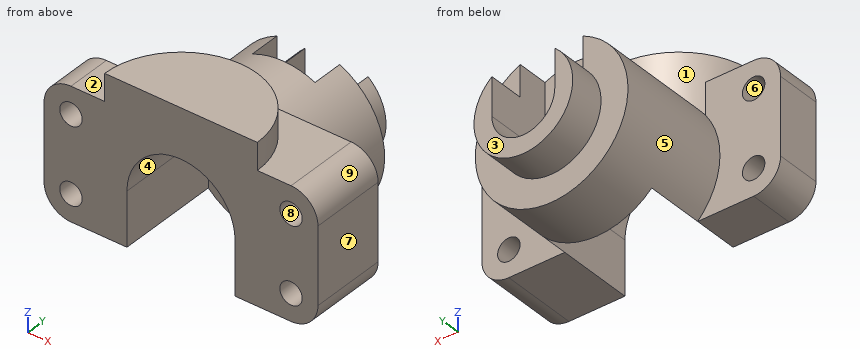
from build123d import *

# Parameters (mm, degrees)
SKETCH_2_R          = 17
EXTRUDE_1_DEPTH     = 36
EXTRUDE_3_REACH     = 52.14
SKETCH_4_R          = 11
SKETCH_5_R          = 7
CUT_EXTRUDE_1_DEPTH = 21
SKETCH_6_W          = 14
SKETCH_6_H          = 15
CUT_EXTRUDE_2_DEPTH = 21
EXTRUDE_5_DEPTH     = 23
SKETCH_8_R          = 2.5
EXTRUDE_6_DEPTH     = 17
SKETCH_9_R          = 2.5
EXTRUDE_7_DEPTH     = 10
CUT_EXTRUDE_3_DEPTH = 23


with BuildPart() as part:
    # 草图2 → 凸台-拉伸1 (new body)
    with BuildSketch(Plane(origin=(0, 0, 0), x_dir=(1, 0, 0), z_dir=(0, 1, 0))):
        with Locations(Location((0, 0, 0), (0, 0, 270))):
            Circle(SKETCH_2_R)
    extrude(amount=EXTRUDE_1_DEPTH)

    # 草图4 → 凸台-拉伸3 (add, up to next)
    with BuildSketch(Plane(origin=(0, 44, 0), x_dir=(1, 0, 0), z_dir=(0, 1, 0)), mode=Mode.PRIVATE) as extrude_3_sk1:
        with Locations(Location((0, 0, 0), (0, 0, 270))):
            Circle(SKETCH_4_R)
    extrude_3_tool1 = extrude(extrude_3_sk1.sketch, amount=-EXTRUDE_3_REACH, mode=Mode.PRIVATE) - part.part
    add(extrude_3_tool1.solids().sort_by_distance((0, 44, 0))[0])

    # 草图5 → 切除-拉伸1 (cut)
    with BuildSketch(Plane(origin=(0, 44, 0), x_dir=(1, 0, 0), z_dir=(0, 1, 0))):
        with Locations(Location((0, 0, 0), (0, 0, 270))):
            Circle(SKETCH_5_R)
    extrude(amount=-CUT_EXTRUDE_1_DEPTH, mode=Mode.SUBTRACT)

    # 草图6 → 切除-拉伸2 (cut)
    with BuildSketch(Plane.XY):
        with Locations((0, 36.5)):
            Rectangle(SKETCH_6_W, SKETCH_6_H)
    extrude(amount=CUT_EXTRUDE_2_DEPTH, mode=Mode.SUBTRACT)

    # 草图7 → 凸台-拉伸5 (add)
    with BuildSketch(Plane.XY.offset(23)):
        with BuildLine():
            Line((-17, 0), (17, 0))
            ThreePointArc((17, 0), (0, 17), (-17, 0))
        make_face()
    extrude(amount=-EXTRUDE_5_DEPTH)

    # 草图8 → 凸台-拉伸6 (add)
    with BuildSketch(Plane(origin=(0, 0, 0), x_dir=(1, 0, 0), z_dir=(0, 1, 0))):
        with BuildLine():
            Line((0, 12), (0, -17))
            Line((0, -17), (24.5, -17))
            ThreePointArc((24.5, -17), (28.742640687, -15.242640687), (30.5, -11))
            Line((30.5, -11), (30.5, 6))
            ThreePointArc((30.5, 6), (28.742640687, 10.242640687), (24.5, 12))
            Line((24.5, 12), (0, 12))
        make_face()
        with Locations(Location((24.5, 6, 0), (0, 0, 270))):
            Circle(SKETCH_8_R, mode=Mode.SUBTRACT)
        with Locations(Location((24.5, -11, 0), (0, 0, 270))):
            Circle(SKETCH_8_R, mode=Mode.SUBTRACT)
    extrude(amount=EXTRUDE_6_DEPTH)

    # 草图9 → 凸台-拉伸7 (add)
    with BuildSketch(Plane(origin=(0, 0, 0), x_dir=(1, 0, 0), z_dir=(0, 1, 0))):
        with BuildLine():
            Line((0, 12), (0, -17))
            Line((0, -17), (-24.5, -17))
            ThreePointArc((-24.5, -17), (-28.742640687, -15.242640687), (-30.5, -11))
            Line((-30.5, -11), (-30.5, 6))
            ThreePointArc((-30.5, 6), (-28.742640687, 10.242640687), (-24.5, 12))
            Line((-24.5, 12), (0, 12))
        make_face()
        with Locations(Location((-24.5, 6, 0), (0, 0, 270))):
            Circle(SKETCH_9_R, mode=Mode.SUBTRACT)
        with Locations(Location((-24.5, -11, 0), (0, 0, 270))):
            Circle(SKETCH_9_R, mode=Mode.SUBTRACT)
    extrude(amount=EXTRUDE_7_DEPTH)

    # 草图10 → 切除-拉伸3 (cut)
    with BuildSketch(Plane(origin=(0, 0, 0), x_dir=(1, 0, 0), z_dir=(0, 1, 0))):
        with BuildLine():
            Line((-12.041594579, 12), (-12.041594579, 0))
            ThreePointArc((-12.041594579, 0), (0, -12.041594579), (12.041594579, 0))
            Line((12.041594579, 0), (12.041594579, 12))
            ThreePointArc((12.041594579, 12), (0, 17), (-12.041594579, 12))
        make_face()
    extrude(amount=CUT_EXTRUDE_3_DEPTH, mode=Mode.SUBTRACT)


solid = part.part
Verification items for the finished model (mm, model axes). Face numbers are marked on the shaded views. A direction names the side the tool comes from. Give positions to 0.01 mm unless a question says otherwise; leave off trailing zeros. Write each loop counter-clockwise with the first axis right and the second up, starting at its lowest first coordinate (ties: lowest second). Pieces come first, ordered by that corner, then holes. Notation, with made-up numbers: M -24,74 L 21,74 A25 ccw 21,102 Z; hole C 7.25,87 d7. An arc over 180 degrees is marked long. Put each result on its own line as item: value. Start each with the question number.
1. Section check A-A (y = 6). Record the cut outline in (x, z).
2. Go/stop test with flat-tipped pins: pin 1 Ø19.5 at (x, z) = (-1, -8.5) entering from -Y; pin 2 Ø3 at (y, z) = (36.5, -3) entering from +X; pin 3 Ø4 at (y, z) = (38.5, 14) entering from -X; pin 4 Ø6 at (x, z) = (-24.5, -6) entering from +Y. Record where each tip stops, or that it passes through.
3. Scan lines: line 1 along X through (y, z) = (3, -6); line 2 along Z through (x, y) = (-24, 5); line 3 along X through (y, z) = (13, 11). Record each from-to range of solid material in increasing order. Write a range as [from, to].
4. Section check B-B (x = 1.5). Record the cut outline in (y, z).
5. Section check D-D (z = 19.5). Record the cut outline in (x, y), and give its area (3 significant figures).
6. Section check C-C (z = -1). Record the cut outline in (x, y).
7. Set-up check for the marked faces 1, 2, 3, 4 and 5: record each of +Z, -Z, +X, -X, +Y, -Y from which the full face is reachable in a straight line by a thin tool's end or side.
8. Draft check along Z on the marked faces 6, 7, 8 and 9. Enter one of: +Z half, -Z half, draft (parallel to the pull), parting line (faces both ways), or undercut.
Answer list:
1. outline: M -30.5,-6 A6 ccw -24.5,-12 L -12.04,-12 L -12.04,0 A12.04 cw 12.04,0 L 12.04,-12 L 24.5,-12 A6 ccw 30.5,-6 L 30.5,11 A6 ccw 24.5,17 L 15.91,17 L 15.91,23 L -15.91,23 L -15.91,17 L -24.5,17 A6 ccw -30.5,11 Z; hole C -24.5,-6 d5; hole C -24.5,11 d5; hole C 24.5,-6 d5; hole C 24.5,11 d5
2. pin 1: y = 23
2. pin 2: x = 16.93
2. pin 3: through
2. pin 4: y = 10
3. line 1: [-30.5, -27], [-22, -12.04], [12.04, 22], [27, 30.5]
3. line 2: [-12, -8.45], [-3.55, 8.55], [13.45, 17]
3. line 3: [-12.96, -4.9], [4.9, 22], [27, 30.5]
4. outline: M 0,11.95 L 23,11.95 L 23,6.84 L 29,6.84 L 29,16.93 L 17,16.93 L 17,17 L 16.93,17 L 16.93,23 L 0,23 Z; M 23,-16.93 L 36,-16.93 L 36,-10.9 L 44,-10.9 L 44,-6.84 L 23,-6.84 Z
5. outline: M -17,0 L 17,0 A17 ccw Z
5. area: 454 mm2
6. outline: M -30.5,0 L -12.04,0 L -12.04,23 L -6.93,23 L -6.93,44 L -10.95,44 L -10.95,36 L -16.97,36 L -16.97,10 L -30.5,10 Z; M 6.93,23 L 12.04,23 L 12.04,0 L 30.5,0 L 30.5,17 L 16.97,17 L 16.97,36 L 10.95,36 L 10.95,44 L 6.93,44 Z
7. face 1: +Z, +Y
7. face 2: +Z, -X, +Y
7. face 3: +Z, -Z, +X, -X, +Y
7. face 4: -Z, -Y
7. face 5: +Y
8. face 6: undercut
8. face 7: draft
8. face 8: undercut
8. face 9: +Z half
